```python
from build123d import *

# Parameters (mm, degrees)
SKETCH1_W               = 150
SKETCH1_H               = 90
BOSS_EXTRUDE1_DEPTH     = 70
SHELL4_T                = -5
SKETCH2_R               = 20
BOSS_EXTRUDE2_DEPTH     = 2.5
SKETCH3_R               = 7.5
BOSS_EXTRUDE3_DEPTH     = 35
SKETCH4_W               = 65
SKETCH4_H               = 4.658499389
CUT_EXTRUDE1_DEPTH      = 189.414436814
SKETCH6_W               = 3
SKETCH6_H               = 3
CUT_EXTRUDE3_DEPTH      = 40
FILLET4_R               = 5
FILLET5_R               = 5
SKETCH10_W              = 3
SKETCH10_H              = 3
CUT_EXTRUDE4_DEPTH      = 40
CUT_EXTRUDE5_DEPTH      = 187.614576065
CUT_EXTRUDE5_DEPTH_BACK = 187.614576065
SKETCH11_W              = 3
SKETCH11_H              = 3
SKETCH11_R              = 20
SKETCH12_W              = 30
SKETCH12_H              = 10
BOSS_EXTRUDE4_DEPTH     = 7.5
CUT_EXTRUDE8_DEPTH      = 146.17231141
CUT_EXTRUDE8_DEPTH_BACK = 146.17231141


with BuildPart() as part:
    # Sketch1 → Boss-Extrude1 (new body)
    with BuildSketch(Plane.XY):
        with Locations((75, -45)):
            Rectangle(SKETCH1_W, SKETCH1_H)
    extrude(amount=BOSS_EXTRUDE1_DEPTH)

    # Shell4
    shell4_openings = [part.faces().sort_by_distance(p)[0] for p in [
        (75, -45, 70),
    ]]
    offset(amount=SHELL4_T, openings=shell4_openings, kind=Kind.INTERSECTION)

    # Sketch2 → Boss-Extrude2 (add)
    with BuildSketch(Plane.XY.offset(5)):
        with Locations((45, -45)):
            Circle(SKETCH2_R)
        with Locations((105, -45)):
            Circle(SKETCH2_R)
    extrude(amount=BOSS_EXTRUDE2_DEPTH)

    # Sketch3 → Boss-Extrude3 (add)
    with BuildSketch(Plane.XY.offset(7.5)):
        with Locations((45, -45)):
            Circle(SKETCH3_R)
        with Locations((105, -45)):
            Circle(SKETCH3_R)
    extrude(amount=BOSS_EXTRUDE3_DEPTH)

    # Sketch4 → Cut-Extrude1 (cut, through all)
    with BuildSketch(Plane.XZ.offset(90)):
        Polygon((85, 70), (85, 49.954434269), (85, 34.954434269), (150, 34.954434269), (150, 70), align=None)
        with Locations((117.5, 72.329249694)):
            Rectangle(SKETCH4_W, SKETCH4_H)
    extrude(amount=-CUT_EXTRUDE1_DEPTH, mode=Mode.SUBTRACT)

    # Sketch6 → Cut-Extrude3 (cut)
    with BuildSketch(Plane.XY.offset(34.954434269)):
        with Locations((96.5, -2.5)):
            Rectangle(SKETCH6_W, SKETCH6_H)
        with Locations((113.5, -2.5)):
            Rectangle(SKETCH6_W, SKETCH6_H)
        with Locations((96.5, -87.5)):
            Rectangle(SKETCH6_W, SKETCH6_H)
        with Locations((113.5, -87.5)):
            Rectangle(SKETCH6_W, SKETCH6_H)
    extrude(amount=-CUT_EXTRUDE3_DEPTH, mode=Mode.SUBTRACT)

    # Fillet4
    fillet4_edges = [part.edges().sort_by_distance(p)[0] for p in [
        (5, -5, 37.5),
        (5, -85, 37.5),
        (145, -5, 19.977217134),
        (145, -85, 19.977217134),
        (150, 0, 17.477217134),
        (150, -90, 17.477217134),
        (85, -87.5, 70),
        (85, -87.5, 34.954434269),
        (85, -2.5, 70),
        (85, -2.5, 34.954434269),
        (0, 0, 35),
        (0, -90, 35),
    ]]
    fillet(fillet4_edges, radius=FILLET4_R)

    # Fillet5
    fillet5_edges = [part.edges().sort_by_distance(p)[0] for p in [
        (37.5, -45, 42.5),
        (97.5, -45, 34.954434269),
    ]]
    fillet(fillet5_edges, radius=FILLET5_R)

    # Sketch10 → Cut-Extrude4 (cut)
    with BuildSketch(Plane.XY.offset(70)):
        with Locations((2.5, -45)):
            Rectangle(SKETCH10_W, SKETCH10_H)
        with Locations((37.5, -87.5)):
            Rectangle(SKETCH10_W, SKETCH10_H)
        with Locations((37.5, -2.5)):
            Rectangle(SKETCH10_W, SKETCH10_H)
    extrude(amount=-CUT_EXTRUDE4_DEPTH, mode=Mode.SUBTRACT)

    # Sketch11 → Cut-Extrude5 (cut, two sides: drawn at the far end of the back side and taken through both)
    # profile 1 of 4: a face of its own
    with BuildSketch(Plane.XY.offset(5).offset(-CUT_EXTRUDE5_DEPTH_BACK)):
        with BuildLine():
            Line((85, -5), (85, 0))
            Line((85, 0), (80, 0))
            Line((80, 0), (5, 0))
            ThreePointArc((5, 0), (1.464466094, -1.464466094), (0, -5))
            Line((0, -5), (0, -85))
            ThreePointArc((0, -85), (1.464466094, -88.535533906), (5, -90))
            Line((5, -90), (80, -90))
            Line((80, -90), (85, -90))
            Line((85, -90), (85, -85))
            Line((85, -85), (80, -85))
            Line((80, -85), (10, -85))
            ThreePointArc((10, -85), (6.464466094, -83.535533906), (5, -80))
            Line((5, -80), (5, -10))
            ThreePointArc((5, -10), (6.464466094, -6.464466094), (10, -5))
            Line((10, -5), (80, -5))
            Line((80, -5), (85, -5))
        make_face()
        with Locations((37.5, -87.5)):
            Rectangle(SKETCH11_W, SKETCH11_H, mode=Mode.SUBTRACT)
        with Locations((2.5, -45)):
            Rectangle(SKETCH11_W, SKETCH11_H, mode=Mode.SUBTRACT)
        with Locations((37.5, -2.5)):
            Rectangle(SKETCH11_W, SKETCH11_H, mode=Mode.SUBTRACT)
    # profile 2 of 4: a face of its own
    with BuildSketch(Plane.XY.offset(5).offset(-CUT_EXTRUDE5_DEPTH_BACK)):
        with BuildLine():
            ThreePointArc((140, -85), (143.535533906, -83.535533906), (145, -80))
            Line((145, -80), (145, -10))
            ThreePointArc((145, -10), (143.535533906, -6.464466094), (140, -5))
            Line((140, -5), (10, -5))
            ThreePointArc((10, -5), (6.464466094, -6.464466094), (5, -10))
            Line((5, -10), (5, -80))
            ThreePointArc((5, -80), (6.464466094, -83.535533906), (10, -85))
            Line((10, -85), (140, -85))
        make_face()
        with Locations((105, -45)):
            Circle(SKETCH11_R, mode=Mode.SUBTRACT)
        with Locations((45, -45)):
            Circle(SKETCH11_R, mode=Mode.SUBTRACT)
    # profile 3 of 4: a face of its own
    with BuildSketch(Plane.XY.offset(5).offset(-CUT_EXTRUDE5_DEPTH_BACK)):
        with BuildLine():
            Line((145, 0), (90, 0))
            Line((90, 0), (85, 0))
            Line((85, 0), (85, -5))
            Line((85, -5), (90, -5))
            Line((90, -5), (140, -5))
            ThreePointArc((140, -5), (143.535533906, -6.464466094), (145, -10))
            Line((145, -10), (145, -80))
            ThreePointArc((145, -80), (143.535533906, -83.535533906), (140, -85))
            Line((140, -85), (90, -85))
            Line((90, -85), (85, -85))
            Line((85, -85), (85, -90))
            Line((85, -90), (90, -90))
            Line((90, -90), (145, -90))
            ThreePointArc((145, -90), (148.535533906, -88.535533906), (150, -85))
            Line((150, -85), (150, -5))
            ThreePointArc((150, -5), (148.535533906, -1.464466094), (145, 0))
        make_face()
    # profile 4 of 4: a face of its own
    with BuildSketch(Plane.XY.offset(5).offset(-CUT_EXTRUDE5_DEPTH_BACK)):
        with Locations((2.5, -45)):
            Rectangle(SKETCH11_W, SKETCH11_H)
    extrude(amount=CUT_EXTRUDE5_DEPTH + CUT_EXTRUDE5_DEPTH_BACK, mode=Mode.SUBTRACT)


with BuildPart() as cut_extrude5_piece_1:
    # of the separate pieces the step leaves, piece 1, a body of its own (cut_extrude5_pieces_kept)
    add(part.part.solids().sort_by_distance((65, -45, 7.5))[0])



with BuildPart() as cut_extrude5_piece_2:
    # of the separate pieces the step leaves, piece 2, a body of its own (cut_extrude5_pieces_kept)
    add(part.part.solids().sort_by_distance((112.5, -45, 29.954434269))[0])


with BuildPart() as cut_extrude5_piece_1_1:
    add(cut_extrude5_piece_1.part)

    add(cut_extrude5_piece_2.part)  # Boss-Extrude4 merges Cut-Extrude5 piece 2
    # Sketch12 → Boss-Extrude4 (add)
    with BuildSketch(Plane.XY.offset(7.5)):
        with Locations((75, -45)):
            Rectangle(SKETCH12_W, SKETCH12_H)
    extrude(amount=-BOSS_EXTRUDE4_DEPTH)

    # Sketch13 → Cut-Extrude8 (cut, two sides: drawn at the far end of the back side and taken through both)
    with BuildSketch(Plane.XY.offset(7.5).offset(-CUT_EXTRUDE8_DEPTH_BACK)):
        with BuildLine():
            ThreePointArc((64.364916731, -40), (25, -45), (64.364916731, -50))
            Line((64.364916731, -50), (53.660254038, -50))
            ThreePointArc((53.660254038, -50), (35, -45), (53.660254038, -40))
            Line((53.660254038, -40), (64.364916731, -40))
        make_face()
        with BuildLine():
            Line((96.339745962, -50), (85.635083269, -50))
            ThreePointArc((85.635083269, -50), (107.52008585, -64.840593925), (125, -45))
            ThreePointArc((125, -45), (107.52008585, -25.159406075), (85.635083269, -40))
            Line((85.635083269, -40), (96.339745962, -40))
            ThreePointArc((96.339745962, -40), (107.588190451, -35.340741737), (115, -45))
            ThreePointArc((115, -45), (107.588190451, -54.659258263), (96.339745962, -50))
        make_face()
    extrude(amount=CUT_EXTRUDE8_DEPTH + CUT_EXTRUDE8_DEPTH_BACK, mode=Mode.SUBTRACT)


solid = cut_extrude5_piece_1_1.part
```
CAD build for the part. Positions are in the model's coordinates, mm. A direction names the side the tool comes from. Round coordinates to 2 decimals unless told otherwise and drop trailing zeros. Order: outer loops, then holes, each group sorted by start corner. A loop starts at its lowest first (then second) coordinate and runs counter-clockwise, first axis right, second up. Notation, with made-up numbers: (54.5, -16.75) - (87.5, -16.75) arc R9 ccw to (87.5, -5.75) - close; hole circle Ø9 at (53.25, -19). An arc over 180 degrees is marked (long way). Answer as CSV lines item,"result". Start each with the question number.
1. Pin check, flat tips, straight feed: pin 1 (5 mm diameter, centred on x = 44.5, z = 34, fed in from +Y); pin 2 (4 mm diameter, centred on x = 65.5, z = 4, fed in from -Y); pin 3 (3 mm diameter, centred on x = 96, z = 5.5, fed in from -Y); pin 4 (12 mm diameter, centred on x = 52.5, y = -44.5, fed in from -Z). Stop position of each tip, or through.
2. Tool access for faces 1 (the face through (75, -50, 4)), 2 (the face through (75, -40, 4)), 3 (the face through (105, -45, 34.954)), 4 (the face through (48.461, -51.654, 22.29)), 5 (the face through (35, -45, 4)): list every direction of +Z, -Z, +X, -X, +Y, -Y with a clear straight run to the whole face (end or side of a thin tool).
3. Saw through at A-A, the plane y = -36.75. Write the cut outline in (x, z), and give its area (3 significant figures).
4. Drill centre lines: L1, parallel to Z at x = 88.5, y = -42.5; L2, parallel to X at y = -45.5, z = 11; L3, parallel to X at y = -41, z = 11.5. Where is each one in solid material? Low to high. Write a range as [from, to].
5. Saw through at C-C, the plane x = 86.5. Write the cut outline in (y, z), and give its area (3 significant figures).
6. Saw through at B-B, the plane z = 14.5. Write the cut outline in (x, y).
Model answer:
1,pin 1,"stops at y = -37.5"
1,pin 2,"stops at y = -50"
1,pin 3,"stops at y = -51.61"
1,pin 4,"stops at z = 0"
2,face 1,"+Z, -Z, -Y"
2,face 2,"+Z, -Z, +Y"
2,face 3,"+Z, +X, +Y, -Y"
2,face 4,"+Z"
2,face 5,"+Z, -Z"
3,outline,"(39.35, 0) - (50.65, 0) - (50.65, 7.5) - (39.35, 7.5) - close; (99.35, 0) - (110.65, 0) - (110.65, 7.5) - (99.35, 7.5) - close"
3,area,"170 mm²"
4,L1,"z = [0, 7.5]"
4,L2,"x = [37.52, 52.48], [97.52, 112.48]"
4,L3,"x = [38.66, 51.34], [98.66, 111.34]"
5,outline,"(-50, 0) - (-40, 0) - (-40, 7.5) - (-50, 7.5) - close"
5,area,"75.0 mm²"
6,outline,"circle Ø15 at (45, -45); circle Ø15 at (105, -45)"
